Drawing for the job (mm, zero at the part's lowest x, y, z). Round coordinates to 2 decimals unless told otherwise and drop trailing zeros. Write each loop counter-clockwise with the first axis right and the second up, starting at its lowest first coordinate (ties: lowest second). Pieces come first, ordered by that corner, then holes. Notation, with made-up numbers: (-28.5, 81.25) - (18.5, 81.25) arc R14 cw to (18.5, 103.25) - close; hole circle Ø5 at (60.5, 47). An arc over 180 degrees is marked (long way). One line per question, with ' | ' between items.
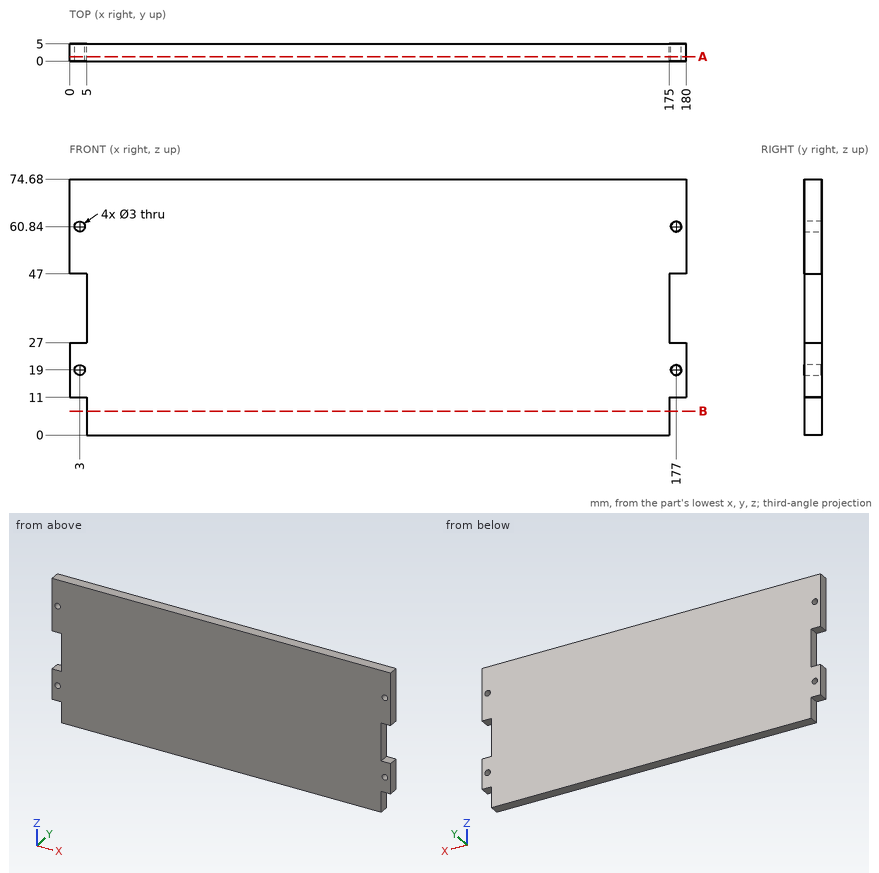
Q1. Saw through at B-B, the plane z = 7. List the corners of the cut face in (x, y), then the cut area to 3 significant figures.
Found:
outline: (5, 0) - (175, 0) - (175, 5) - (5, 5) - close | area: 850 mm^2
Q2. Saw through at A-A, the plane y = 1.35. List the corners of the cut face in (x, z).
Found:
outline: (0, 11) - (5, 11) - (5, 0) - (175, 0) - (175, 11) - (180, 11) - (180, 27) - (175, 27) - (175, 47) - (180, 47) - (180, 74.68) - (0, 74.68) - (0, 47) - (5, 47) - (5, 27) - (0, 27) - close; hole circle Ø3 at (3, 19); hole circle Ø3 at (3, 60.84); hole circle Ø3 at (177, 19); hole circle Ø3 at (177, 60.84)
Q3. Drop flat-ended pins along their axis: pin 1 (8 mm diameter, centred on x = 104.5, z = 39, fed in from -Y); pin 2 (2.5 mm diameter, centred on x = 3, z = 60.84, fed in from -Y); pin 3 (1.5 mm diameter, centred on y = 2.5, z = 38.5, fed in from -X); pin 4 (1.5 mm diameter, centred on x = 2, y = 3.5, fed in from -Z). Give the stop position or say it passes through.
Found:
pin 1: y = 0 | pin 2: through | pin 3: x = 5 | pin 4: z = 11
Q4. Drill centre lines: L1, parallel to X at y = 3.5, z = 60.84; L2, parallel to Z at x = 177, y = 2.45; L3, parallel to X at y = 4.4, z = 36. Where is each one in solid material? Low to high. Write a range as from..to.
Found:
L1: 0..1.5, 4.5..175.5, 178.5..180 | L2: 11..17.5, 20.5..27, 47..59.34, 62.34..74.68 | L3: 5..175
